```python
from build123d import *

# Parameters (mm, degrees)
SKETCH_2_R          = 2.1
EXTRUDE_1_DEPTH     = 2.5
CHAMFER_1_SIZE      = 2
CHAMFER_2_SIZE      = 4
CUT_EXTRUDE_1_DEPTH = 70.641941386


with BuildPart() as part:
    # 草图2 → 凸台-拉伸1 (new, symmetric)
    with BuildSketch(Plane(origin=(0, 0, 0), x_dir=(1, 0, 0), z_dir=(0, 1, 0))):
        Polygon((0, 35), (-10, 35), (-60, -15), (-60, -35), (60, -35), (60, -15), (10, 35), align=None)
        with Locations(Location((-50, -25, 0), (0, 0, 270))):
            Circle(SKETCH_2_R, mode=Mode.SUBTRACT)
        with Locations(Location((0, 25, 0), (0, 0, 270))):
            Circle(SKETCH_2_R, mode=Mode.SUBTRACT)
        with Locations(Location((0, -5, 0), (0, 0, 270))):
            Circle(SKETCH_2_R, mode=Mode.SUBTRACT)
        with Locations(Location((0, -25, 0), (0, 0, 270))):
            Circle(SKETCH_2_R, mode=Mode.SUBTRACT)
        with Locations(Location((50, -25, 0), (0, 0, 90))):
            Circle(SKETCH_2_R, mode=Mode.SUBTRACT)
    extrude(amount=EXTRUDE_1_DEPTH, both=True)

    # 倒角1
    chamfer_1_edges = [part.edges().sort_by_distance(p)[0] for p in [
        (-50, 2.5, 22.9),
        (0, 2.5, -27.1),
        (0, 2.5, 2.9),
        (0, 2.5, 22.9),
        (50, 2.5, 27.1),
    ]]
    chamfer(chamfer_1_edges, length=CHAMFER_1_SIZE)

    # 倒角2
    chamfer_2_edges = [part.edges().sort_by_distance(p)[0] for p in [
        (60, 0, 35),
        (-60, 0, 35),
    ]]
    chamfer(chamfer_2_edges, length=CHAMFER_2_SIZE)

    # 草图3 → 切除-拉伸1 (cut, through all)
    with BuildSketch(Plane(origin=(0, 2.5, 0), x_dir=(1, 0, 0), z_dir=(0, 1, 0))):
        with BuildLine():
            Line((-30.251262658, -6.464466094), (-18.535533906, 5.251262658))
            ThreePointArc((-18.535533906, 5.251262658), (-11.464466094, 5.251262658), (-11.464466094, -1.819805153))
            Line((-11.464466094, -1.819805153), (-23.180194847, -13.535533906))
            ThreePointArc((-23.180194847, -13.535533906), (-30.251262658, -13.535533906), (-30.251262658, -6.464466094))
        make_face()
        with BuildLine():
            Line((30.251262658, -6.464466094), (18.535533906, 5.251262658))
            ThreePointArc((18.535533906, 5.251262658), (11.464466094, 5.251262658), (11.464466094, -1.819805153))
            Line((11.464466094, -1.819805153), (23.180194847, -13.535533906))
            ThreePointArc((23.180194847, -13.535533906), (30.251262658, -13.535533906), (30.251262658, -6.464466094))
        make_face()
    extrude(amount=-CUT_EXTRUDE_1_DEPTH, mode=Mode.SUBTRACT)


solid = part.part
```
Design review of the part built by this model. Coordinates are the model's own, in mm. A direction names the side the tool comes from. Give positions to 0.01 mm unless a question says otherwise; leave off trailing zeros. Order: outer loops, then holes, each group sorted by start corner. A loop starts at its lowest first (then second) coordinate and runs counter-clockwise, first axis right, second up. Notation, with made-up numbers: (-20, 44) - (15, 44) arc R32 cw to (15, 75) - close; hole circle Ø8 at (56.5, 83). An arc over 180 degrees is marked (long way). Use a Markdown table: item, result. Add a question column.
(1) Clearance check with flat-ended pins moving along their axes: P1, Ø5, axis at x = 0, z = -25, coming from the +Y side; P2, Ø5.5, axis at x = 0, z = 5, coming from the +Y side; P3, Ø2, axis at y = -2, z = -3, coming from the -X side. State where each tip first meets the part, or that it passes through.
(2) Add section B-B on z = -25. Give the boundary of the cut face in (x, y).
(3) Add section D-D on x = 0. Give the boundary of the cut face in (y, z).
(4) Wall thickness on probe 1 along X at (y, z) = (-0.6, 25); probe 2 along X at (y, z) = (-0.75, 5); probe 3 along X at (y, z) = (-2.05, 10): over which ranges is each line inside the solid? List them lowest first. Write a range as [from, to].
(5) Add section A-A on x = 50. Give the boundary of the cut face in (y, z), then the cut area to 3 significant figures.
(6) Add section C-C on y = 1.55. Give the boundary of the cut face in (x, z).
(7) Machinability: for faces 1 (the face through (-1, 2.5, 15)), 2 (the face through (-17.24, 0.035, 7.596)), which of the approach directions +Z, -Z, +X, -X, +Y, -Y give a long, thin tool a straight path to every point of the face, cutting with its end or side? Answer none if there is none.
(8) Mouldability with a two-part tool opening along Z and no side actions: class faces 3 (the face through (35, 0, -10)), 4 (the face through (11.543, 0.035, -5.328)), 5 (the face through (-60, 0, 23)) as +Z half, -Z half, draft (parallel to the pull), parting line (faces both ways), or undercut.
Report:
| question | item | result |
|---|---|---|
| 1 | P1 | stops at y = 0.9 |
| 1 | P2 | stops at y = 1.15 |
| 1 | P3 | stops at x = -43 |
| 2 | outline | (-20, -2.5) - (-2.1, -2.5) - (-2.1, 0.5) - (-4.1, 2.5) - (-20, 2.5) - close; (2.1, -2.5) - (20, -2.5) - (20, 2.5) - (4.1, 2.5) - (2.1, 0.5) - close |
| 3 | outline | (-2.5, -35) - (2.5, -35) - (2.5, -29.1) - (0.5, -27.1) - (-2.5, -27.1) - close; (-2.5, -22.9) - (0.5, -22.9) - (2.5, -20.9) - (2.5, 0.9) - (0.5, 2.9) - (-2.5, 2.9) - close; (-2.5, 7.1) - (0.5, 7.1) - (2.5, 9.1) - (2.5, 20.9) - (0.5, 22.9) - (-2.5, 22.9) - close; (-2.5, 27.1) - (0.5, 27.1) - (2.5, 29.1) - (2.5, 35) - (-2.5, 35) - close |
| 4 | probe 1 | x = [-60, -52.1], [-47.9, -2.1], [2.1, 47.9], [52.1, 60] |
| 4 | probe 2 | x = [-50, -28.79], [-14.64, -2.1], [2.1, 14.64], [28.79, 50] |
| 4 | probe 3 | x = [-55, -31.72], [-19.64, 19.64], [31.72, 55] |
| 5 | outline | (-2.5, 5) - (2.5, 5) - (2.5, 20.9) - (0.5, 22.9) - (-2.5, 22.9) - close; (-2.5, 27.1) - (0.5, 27.1) - (2.5, 29.1) - (2.5, 35) - (-2.5, 35) - close |
| 5 | area | 125 mm² |
| 6 | outline | (-60, 15) - (-10, -35) - (10, -35) - (60, 15) - (60, 31) - (56, 35) - (-56, 35) - (-60, 31) - close; hole circle Ø6.3 at (-50, 25); hole (-30.25, 6.46) - (-18.54, -5.25) arc R5 ccw to (-11.46, 1.82) - (-23.18, 13.54) arc R5 ccw to start; hole circle Ø6.3 at (0, -25); hole circle Ø6.3 at (0, 5); hole circle Ø6.3 at (0, 25); hole (11.46, 1.82) arc R5 ccw to (18.54, -5.25) - (30.25, 6.46) arc R5 ccw to (23.18, 13.54) - close; hole circle Ø6.3 at (50, 25) |
| 7 | face 1 | +Z, -Z, +X, -X, +Y |
| 7 | face 2 | +Y, -Y |
| 8 | face 3 | -Z half |
| 8 | face 4 | undercut |
| 8 | face 5 | draft |
